```python
from build123d import *

# Parameters (mm, degrees)
F1_DEPTH = 10
F2_R     = 12.5
F3_DEPTH = 10.001
F4_R     = 1


with BuildPart() as f1:
    # F0 (on Front) → F1 (new body)
    with BuildSketch(Plane.XZ):
        Polygon((17.5, 10.10363), (0, 20.207259), (-17.5, 10.10363), (-17.5, -10.10363), (0, -20.207259), (17.5, -10.10363), align=None)
    extrude(amount=F1_DEPTH)

    # F2 (on face) → F3 (cut, through all)
    with BuildSketch(Plane.XZ.offset(10)):
        Circle(F2_R)
    extrude(amount=-F3_DEPTH, mode=Mode.SUBTRACT)

    # F4
    f4_edges = [f1.edges().sort_by_distance(p)[0] for p in [
        (8.75, -10, 15.155445),
        (-8.75, -10, 15.155445),
        (17.5, -10, 0),
        (8.75, -10, -15.155445),
        (-8.75, -10, -15.155445),
        (-17.5, -10, 0),
        (8.75, 0, 15.155445),
        (-8.75, 0, 15.155445),
        (-17.5, 0, 0),
        (-8.75, 0, -15.155445),
        (8.75, 0, -15.155445),
        (17.5, 0, 0),
    ]]
    fillet(f4_edges, radius=F4_R)


solid = f1.part
```
The model under review builds one solid part; all positions refer to its coordinate system, in mm. Coordinates: 2 decimals unless noted, no trailing zeros. Write each loop counter-clockwise with the first axis right and the second up, starting at its lowest first coordinate (ties: lowest second). Pieces come first, ordered by that corner, then holes.
1) We need section B-B on z = 0. State the section outline as (x, y) points, then the cut area to 3 significant figures.
2) Clearance check with flat-ended pins moving along their axes: pin 1 Ø3 at (x, y) = (11, -2) entering from -Z; pin 2 Ø2 at (x, y) = (-8.5, -2) entering from -Z; pin 3 Ø20 at (x, z) = (0, 0) entering from -Y. State where each tip first meets the part, or that it passes through.
3) We need section A-A on y = -3.75. State the section outline as (x, z) points.
4) To check wall thickness, follow probe 1 along Z at (x, y) = (0, -5.75); probe 2 along Z at (x, y) = (-9, -7.5); probe 3 along X at (y, z) = (-0.5, -1.5). State the ranges of each line that lie inside material, in increasing order.
5) The part is to be moulded in two halves that separate along Z. For faces 1 (the face through (11.923, -5.07, 3.755)), 2 (the face through (8.48, -9.7, 14.98)), 3 (the face through (-17.199, -9.715, -0.141)), 4 (the face through (-8.872, -4.944, -15.085)), say which applies: pulls with the +Z half, pulls with the -Z half, needs draft (parallel to the pull), parting line crosses it, or undercut.
Answer list:
1. outline: (-17.5, -9) arc R1 ccw to (-16.5, -10) - (-12.5, -10) - (-12.5, 0) - (-16.5, 0) arc R1 ccw to (-17.5, -1) - close; (12.5, -10) - (16.5, -10) arc R1 ccw to (17.5, -9) - (17.5, -1) arc R1 ccw to (16.5, 0) - (12.5, 0) - close
1. area: 99.1 mm2
2. pin 1: stops at z = -14.72
2. pin 2: stops at z = -15.88
2. pin 3: passes through
3. outline: (-17.5, -10.1) - (0, -20.21) - (17.5, -10.1) - (17.5, 10.1) - (0, 20.21) - (-17.5, 10.1) - close; hole circle Ø25 at (0, 0)
4. probe 1: z = -20.21 to -12.5, 12.5 to 20.21
4. probe 2: z = -15.01 to -8.67, 8.67 to 15.01
4. probe 3: x = -17.37 to -12.41, 12.41 to 17.37
5. face 1: undercut
5. face 2: pulls with the +Z half
5. face 3: needs draft
5. face 4: pulls with the -Z half
